Read the model definition and answer for the solid it produces. Units are mm, in the model's axes. A direction names the side the tool comes from. Give positions to 0.01 mm unless a question says otherwise; leave off trailing zeros. Write each loop counter-clockwise with the first axis right and the second up, starting at its lowest first coordinate (ties: lowest second). Pieces come first, ordered by that corner, then holes. Notation, with made-up numbers: M 65.25,-5 L 110.25,-5 A35 ccw 110.25,34 Z; hole C 68.25,65.5 d9. An arc over 180 degrees is marked long. Use a Markdown table: item, result. Add a question column.
Item 1: Given P1, Ø4, axis at y = 7, z = 0, coming from the -X side; P2, Ø1.5, axis at x = 1, y = 2.5, coming from the +Z side; P3, Ø1, axis at x = 1.5, z = -4, coming from the -Y side; P4, Ø1, axis at x = 5, y = -6, coming from the -Z side, each flat-ended and moving along its own axis, determine where each tip first touches the part or whether it passes through.
Item 2: A cutting plane is placed at A-A on y = -1.5. Determine the outline of the cut face in (x, z), then the cut area to 3 significant figures.
Item 3: For faces 4 (the cylindrical face through (4.93, 10.23, -3.86)), 5 (the cylindrical face through (4.93, -5.28, -9.58)), 6 (the cylindrical face through (4.93, -10.23, 3.86)), determine the directions among +Z, -Z, +X, -X, +Y, -Y from which every point of the face is accessible in a straight line to the end or side of a thin tool.
Item 4: A cutting plane is placed at C-C on x = 9. Count the separate pieces of the cut face and the enclosed holes in it, then the cut area to 3 significant figures.
Item 5: The mould has two halves that part along Y. Classify faces 1 (the cylindrical face through (4.93, -10.206, -3.841)), 2 (the cylindrical face through (4.93, -0.737, 10.912)), 3 (the cylindrical face through (4.93, 10.87, 0.81)): pulls with the +Y half, pulls with the -Y half, needs draft (parallel to the pull), parting line crosses it, or undercut.
Item 6: Consider probe 1 along Y at (x, z) = (4.75, 4); probe 2 along Z at (x, y) = (1.5, -4); probe 3 along Y at (x, z) = (4.5, 9.75). Determine where each line is inside the solid, lowest interval first. Write a range as [from, to].
Item 7: A cutting plane is placed at B-B on z = 0. Determine the outline of the cut face in (x, y).
from build123d import *

# Parameters (mm, degrees)
BASPROSKE_W          = 10
BASPROSKE_H          = 12
TOOTHCUT_DEPTH       = 20.697715604
TEETHCUTS_COUNT      = 22
TEETHCUTS_ANGLE      = 343.636363636
BORSKE_R             = 5
BORE_DEPTH           = 50.0000508
D_GAGEMENT_M21_D     = 2.4
D_GAGEMENT_M21_DEPTH = 10


with BuildPart() as part:
    # BasProSke → Base-Revolve (revolve)
    with BuildSketch(Plane(origin=(0, 0, 0), x_dir=(1, 0, 0), z_dir=(0, 1, 0)), mode=Mode.PRIVATE) as base_revolve_sk:
        with Locations((5, 6)):
            Rectangle(BASPROSKE_W, BASPROSKE_H)
    revolve(base_revolve_sk.sketch.rotate(Axis((-10, 0, 0), (1, 0, 0)), 180), axis=Axis((-10, 0, 0), (1, 0, 0)))

    # TooCutSke → ToothCut (cut, through all)
    with BuildSketch(Plane(origin=(0, 0, 0), x_dir=(0, 0, -1), z_dir=(1, 0, 0))):
        with BuildLine():
            ThreePointArc((0.491001901, 9.736627657), (0, 9.749), (-0.491001901, 9.736627657))
            ThreePointArc((-0.491001901, 9.736627657), (-0.822824844, 10.904005344), (-1.46093845, 11.936327074))
            ThreePointArc((-1.46093845, 11.936327074), (0, 12.0254), (1.46093845, 11.936327074))
            ThreePointArc((1.46093845, 11.936327074), (0.822824844, 10.904005344), (0.491001901, 9.736627657))
        make_face()
    toothcut = extrude(amount=TOOTHCUT_DEPTH, mode=Mode.SUBTRACT)

    # TeethCuts: ToothCut ×22 about axis
    teethcuts_axis = Axis((-10, 0, 0), (1, 0, 0))
    for i in range(1, TEETHCUTS_COUNT):
        add(toothcut.rotate(teethcuts_axis, i * TEETHCUTS_ANGLE / (TEETHCUTS_COUNT - 1)), mode=Mode.SUBTRACT)

    # BorSke → Bore (cut, symmetric)
    with BuildSketch(Plane(origin=(0, 0, 0), x_dir=(0, 0, -1), z_dir=(1, 0, 0))):
        with Locations(Location((0, 0, 0), (0, 0, 180))):
            Circle(BORSKE_R)
    extrude(amount=BORE_DEPTH, both=True, mode=Mode.SUBTRACT)

    # Dégagement M21
    with Locations(Plane(origin=(10, 0, 0), x_dir=(0, 0, -1), z_dir=(1, 0, 0))):
        with Locations((0, 7), (4.949747468, 4.949747468), (7, 0), (4.949747468, -4.949747468), (0, -7), (-4.949747468, -4.949747468), (-7, 0), (-4.949747468, 4.949747468), (0, 0)):
            Hole(D_GAGEMENT_M21_D / 2, depth=D_GAGEMENT_M21_DEPTH)


solid = part.part
Filled in:
| question | item | result |
|---|---|---|
| 1 | P1 | x = 0 |
| 1 | P2 | z = 11.59 |
| 1 | P3 | y = -10.85 |
| 1 | P4 | z = -10.24 |
| 2 | outline | M 0,-9.63 L 10,-9.63 L 10,-4.77 L 0,-4.77 Z; M 0,4.77 L 10,4.77 L 10,9.63 L 0,9.63 Z |
| 2 | area | 97.3 mm² |
| 3 | face 4 | +X, -X, +Y |
| 3 | face 5 | -Z, +X, -X |
| 3 | face 6 | +X, -X, -Y |
| 4 | separate pieces | 1 |
| 4 | enclosed holes | 9 |
| 4 | area | 253 mm² |
| 5 | face 1 | pulls with the -Y half |
| 5 | face 2 | undercut |
| 5 | face 3 | pulls with the +Y half |
| 6 | probe 1 | [-10.39, -5.68], [-4.22, -3], [3, 4.22], [5.68, 10.39] |
| 6 | probe 2 | [-8.89, -5.68], [-4.22, -3], [3, 4.22], [5.68, 8.89] |
| 6 | probe 3 | [-6.7, -5.49], [-3.74, -1.93], [-0.9, 0.9], [1.93, 3.74], [5.49, 6.7] |
| 7 | outline | M 0,-9.75 L 10,-9.75 L 10,-8.2 L 0,-8.2 Z; M 0,-5.8 L 10,-5.8 L 10,-5 L 0,-5 Z; M 0,5 L 10,5 L 10,5.8 L 0,5.8 Z; M 0,8.2 L 10,8.2 L 10,9.75 L 0,9.75 Z |
